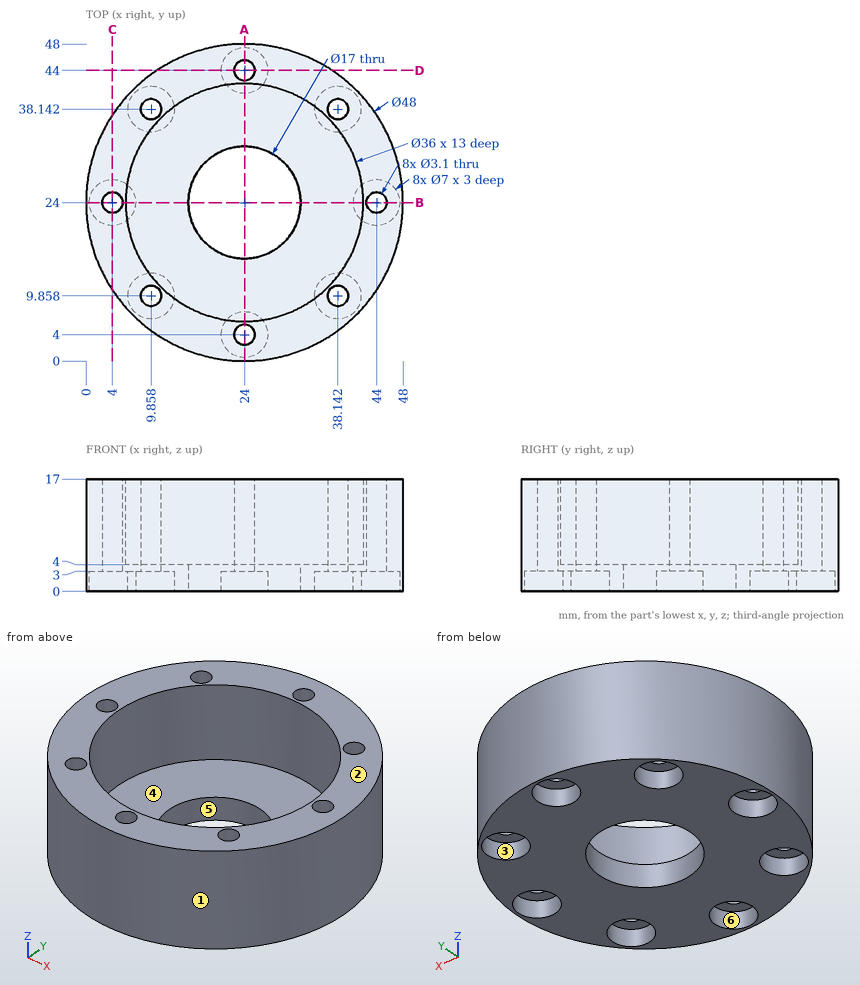
Verification items for this drawing (mm, ordinates from the low corner). A direction names the side the tool comes from. Round coordinates to 2 decimals unless told otherwise and drop trailing zeros. Order: outer loops, then holes, each group sorted by start corner. A loop starts at its lowest first (then second) coordinate and runs counter-clockwise, first axis right, second up. Notation, with made-up numbers: M -8.75,8.25 L 14.25,8.25 A23 ccw 14.25,46.25 Z; hole C 48,25.5 d5. An arc over 180 degrees is marked long. Answer in a Markdown table with one row per item. Add a question column.
Item 1: Set-up check for the marked faces 4, 5 and 6: record each of +Z, -Z, +X, -X, +Y, -Y from which the full face is reachable in a straight line by a thin tool's end or side.
Item 2: Material ranges on L1, parallel to Y at x = 24, z = 2.35; L2, parallel to X at y = 37.5, z = 15.75 (1 decimal); L3, parallel to X at y = 23, z = 1.5, recorded low to high. Write a range as [from, to].
Item 3: Draft check along X on the marked faces 1, 2 and 3. Enter one of: released by +X, released by -X, zero draft, split by the parting line, or undercut.
Item 4: Sectioned sample at C-C, the plane x = 4. Enter the section's corners in (y, z).
Item 5: Sectioned sample at A-A, the plane x = 24. Enter the section's corners in (y, z).
Item 6: Depth check by flat-ended pin: pin 1 Ø15.5 at (x, y) = (24, 24) entering from +Z; pin 2 Ø4 at (x, y) = (9.86, 9.86) entering from -Z; pin 3 Ø2 at (x, z) = (18.5, 14) entering from -Y; pin 4 Ø1.5 at (x, z) = (21, 9.5) entering from -Y. Enter the tip coordinate at first touch or a pass-through.
Filled in:
| question | item | result |
|---|---|---|
| 1 | face 4 | +Z |
| 1 | face 5 | +Z, -Z |
| 1 | face 6 | -Z |
| 2 | L1 | y = [0, 0.5], [7.5, 15.5], [32.5, 40.5], [47.5, 48] |
| 2 | L2 | x = [4.2, 8.4], [11.3, 12.1], [35.9, 36.7], [39.6, 43.8] |
| 2 | L3 | x = [0.02, 0.65], [7.35, 15.56], [32.44, 40.65], [47.35, 47.98] |
| 3 | face 1 | split by the parting line |
| 3 | face 2 | zero draft |
| 3 | face 3 | undercut |
| 4 | outline | M 10.73,0 L 20.5,0 L 20.5,3 L 22.45,3 L 22.45,17 L 10.73,17 Z; M 25.55,3 L 27.5,3 L 27.5,0 L 37.27,0 L 37.27,17 L 25.55,17 Z |
| 5 | outline | M 0,0 L 0.5,0 L 0.5,3 L 2.45,3 L 2.45,17 L 0,17 Z; M 5.55,3 L 7.5,3 L 7.5,0 L 15.5,0 L 15.5,4 L 6,4 L 6,17 L 5.55,17 Z; M 32.5,0 L 40.5,0 L 40.5,3 L 42.45,3 L 42.45,17 L 42,17 L 42,4 L 32.5,4 Z; M 45.55,3 L 47.5,3 L 47.5,0 L 48,0 L 48,17 L 45.55,17 Z |
| 6 | pin 1 | passes through |
| 6 | pin 2 | stops at z = 3 |
| 6 | pin 3 | stops at y = 0.43 |
| 6 | pin 4 | stops at y = 0.11 |
